The listing builds one solid part. Answer for the finished solid, in the listing's coordinates (mm). Face numbers are marked on the shaded views. A direction names the side the tool comes from. Round coordinates to 2 decimals unless told otherwise and drop trailing zeros. Loops run counter-clockwise (first coordinate to the right, second up) from the corner with the lowest first, then second, coordinate; pieces in that order, holes last. Notation, with made-up numbers: (47, 83) -> (89, 83) arc R26 cw to (89, 108) -> close; hole circle Ø10 at (60.25, 83.5). An arc over 180 degrees is marked (long way). One line per question, with ' | ' between items.
from build123d import *

# Parameters (mm, degrees)
F0_W     = 38.1
F0_H     = 38.1
F1_DEPTH = 38.1
F5_DEPTH = 38.1
F7_DEPTH = 38.1
F8_W     = 25.4
F8_H     = 7.62
F9_DEPTH = 38.1


with BuildPart() as f1:
    # F0 (on Front) → F1 (new body)
    with BuildSketch(Plane.XZ):
        with Locations((19.05, 19.05)):
            Rectangle(F0_W, F0_H)
    extrude(amount=F1_DEPTH)

    # F4 (on face) → F5 (cut)
    with BuildSketch(Plane.YZ.offset(38.1)):
        Polygon((-6.35, 38.1), (-31.75, 38.1), (-26.67, 15.875), (-21.59, 25.4), (-16.51, 25.4), (-11.43, 15.875), align=None)
        Polygon((-31.75, 0), (-38.1, 38.1), (-38.1, 0), align=None)
        Polygon((-19.05, 15.875), (-25.4, 0), (-12.7, 0), align=None)
        Polygon((0, 0), (0, 38.1), (-6.35, 0), align=None)
    extrude(amount=-F5_DEPTH, mode=Mode.SUBTRACT)

    # F6 (on offset) → F7 (cut)
    with BuildSketch(Plane.XZ.offset(38.1)):
        Polygon((25.4, 38.1), (12.7, 38.1), (19.05, 22.225), align=None)
        Polygon((6.35, 38.1), (0, 38.1), (0, 0), align=None)
        Polygon((11.43, 22.225), (6.35, 0), (31.75, 0), (26.67, 22.225), (21.59, 9.525), (16.51, 9.525), align=None)
        Polygon((31.75, 38.1), (38.1, 0), (38.1, 38.1), align=None)
    extrude(amount=-F7_DEPTH, mode=Mode.SUBTRACT)

    # F8 (on offset) → F9 (cut)
    with BuildSketch(Plane.XY.offset(38.1)):
        with Locations((12.7, -26.67)):
            Rectangle(F8_W, F8_H)
        with Locations((25.4, -11.43)):
            Rectangle(F8_W, F8_H)
    extrude(amount=-F9_DEPTH, mode=Mode.SUBTRACT)


solid = f1.part
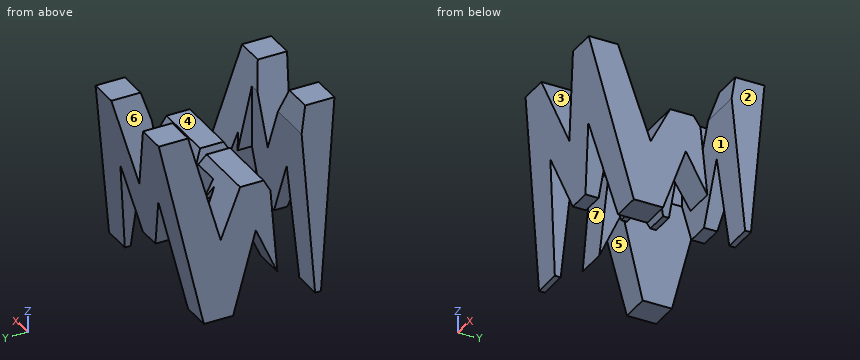
Q1. Given pin 1 Ø3 at (x, y) = (20, -6.5) entering from -Z (3 decimals); pin 2 Ø1.5 at (y, z) = (-4, 14.5) entering from -X; pin 3 Ø12 at (y, z) = (-33.5, 6.5) entering from -X; pin 4 Ø10 at (x, y) = (32.5, -5.5) entering from -Z, each flat-ended and moving along its own axis, determine where each tip first touches the part or whether it passes through.
Numbers:
pin 1: z = 9.525 | pin 2: x = 2.29 | pin 3: x = 0.12 | pin 4: z = 0
Q2. For the marked faces 4, 5, 6 and 7, determine the directions among +Z, -Z, +X, -X, +Y, -Y from which every point of the face is accessible in a straight line to the end or side of a thin tool.
Numbers:
face 4: +Z, +X, -X | face 5: -Z, +X, -X | face 6: +Z, +Y, -Y | face 7: +Z, -Z, -X
Q3. A cutting plane is placed at A-A on z = 30. Give the vertices of the cut face in (x, y).
Numbers:
outline: (5, -36.75) -> (15.94, -36.75) -> (15.94, -30.48) -> (5, -30.48) -> close; (5, -8.2) -> (12.7, -8.2) -> (12.7, -7.62) -> (15.94, -7.62) -> (15.94, -1.35) -> (5, -1.35) -> close; (22.16, -36.75) -> (33.1, -36.75) -> (33.1, -29.9) -> (25.4, -29.9) -> (25.4, -30.48) -> (22.16, -30.48) -> close; (22.16, -7.62) -> (33.1, -7.62) -> (33.1, -1.35) -> (22.16, -1.35) -> close
Q4. A cutting plane is placed at C-C on z = 8. Give the vertices of the cut face in (x, y).
Numbers:
outline: (1.33, -33.08) -> (8.18, -33.08) -> (8.18, -30.48) -> (1.33, -30.48) -> close; (1.33, -22.86) -> (8.18, -22.86) -> (8.18, -22.2) -> (1.33, -22.2) -> close; (1.33, -15.9) -> (8.18, -15.9) -> (8.18, -5.02) -> (1.33, -5.02) -> close; (29.92, -33.08) -> (36.77, -33.08) -> (36.77, -22.2) -> (29.92, -22.2) -> close; (29.92, -15.9) -> (36.77, -15.9) -> (36.77, -15.24) -> (29.92, -15.24) -> close; (29.92, -7.62) -> (36.77, -7.62) -> (36.77, -5.02) -> (29.92, -5.02) -> close
Q5. A cutting plane is placed at B-B on y = -24. Give the vertices of the cut face in (x, z).
Numbers:
outline: (25.4, 19.05) -> (26.13, 20.88) -> (25.4, 20.88) -> close; (26.98, 20.88) -> (30.95, 3.5) -> (37.52, 3.5) -> (34.62, 20.88) -> close
Q6. For a pull along X with two mould halves and no side action, classify the marked faces 1, 2 and 3 as pulls with the +X half, pulls with the -X half, needs draft (parallel to the pull), parting line crosses it, or undercut.
Numbers:
face 1: needs draft | face 2: pulls with the +X half | face 3: undercut
Q7. Find the intervals of material crossed by line 1 (Y direction, x = 9, z = 13); line 2 (X direction, y = -16, z = 18); line 3 (X direction, y = -20, z = 16.5), in increasing order. Write a range as from..to.
Numbers:
line 1: -33.92..-30.48, -22.86..-20.2, -17.9..-4.18 | line 2: 3..10.46, 13.12..24.98, 27.64..35.1 | line 3: 2.75..10.12, 13.72..24.38, 27.98..35.35
